Can you work these out from the model? Positions are in its coordinate system, mm. A direction names the side the tool comes from. Coordinates: 2 decimals unless noted, no trailing zeros. Loops run counter-clockwise (first coordinate to the right, second up) from the corner with the lowest first, then second, coordinate; pieces in that order, holes last. Notation, with made-up numbers: (28.25, -37) - (86.25, -37) arc R22 ccw to (86.25, -3) - close; hole circle Ø9 at (-39.5, -12.75). An arc over 180 degrees is marked (long way). Put each result on its own line as item: value. Start each with the question number.
Solid Edge part; units mm, degrees
sketch "Sketch1" plane through (0, 0, 0) normal (0, 0, 1) x (1, 0, 0)
  circle A0 centre (0, 0) radius 10
extrude "Protrusion1" add sketch "Sketch1" along normal mid plane 11
sketch "Sketch2" plane through (0, 0, 5.5) normal (0, 0, 1) x (0, 1, 0)
  circle A0 centre (0, 0) radius 14.5
extrude "ExtrudedProtrusion_2" add sketch "Sketch2" along normal blind 3
mirror "Mirror1" about plane through (0, 0, 0) normal (0, 0, -1) of "ExtrudedProtrusion_2"
sketch "Sketch3" plane through (0, 0, 8.5) normal (0, 0, 1) x (0, -1, 0)
  line L0 (3.9285, -6.3953) -> (7.5028, 0.2046)
  line L1 (7.5028, 0.2046) -> (3.5742, 6.5999)
  line L2 (3.5742, 6.5999) -> (-3.9285, 6.3953)
  line L3 (-3.9285, 6.3953) -> (-7.5028, -0.2046)
  line L4 (-7.5028, -0.2046) -> (-3.5742, -6.5999)
  line L5 (-3.5742, -6.5999) -> (3.9285, -6.3953)
extrude "ExtrudedCutout_1" cut sketch "Sketch3" against normal blind 37.5006
properties part number "BumbleB0195"
Q1. On a 3-axis mill with a long thin cutter (end or side, diameter ignored), from which of +Z, -Z, +X, -X, +Y, -Y can I reach the whole of each face in a straight line? I mean faces 5 (the flat face through (-3, 10, -5.5)), 6 (the flat face through (-3.14, -5.69, 0.12)), 7 (the flat face through (7, 0, -8.5)). Say none if no direction works.
Q2. I want a section at B-B on z = 4.75. List the corners of the cut face in (x, y) for me.
Q3. Will these pins go through, and if not, where does the flat tip stop? pin 1 (1 mm diameter, centred on x = 3.5, z = -3.5, fed in from +Y); pin 2 (1.5 mm diameter, centred on x = 9.5, z = 1, fed in from +Y); pin 3 (10 mm diameter, centred on x = 6, z = 5.5, fed in from -Y); pin 4 (8.5 mm diameter, centred on x = -1, y = -3, fed in from +Z).
Q4. We'd pull the mould along Z, two halves only. Please class faces 1 (the flat face through (3, 10, 5.5)), 2 (the flat face through (3.14, 5.69, 0.12)), 3 (the cylindrical face through (-2.17, -9.76, 0.08)), 4 (the flat face through (-7, 0, 8.5)): released by +Z, released by -Z, zero draft, split by the parting line, or undercut.
Q5. Please list where these lines run through material, in increasing order: line 1 along Z through (x, y) = (-10.75, 6); line 2 along X through (y, z) = (7.25, -0.5); line 3 along Y through (x, z) = (4.5, -4). Write a range as [from, to].
Q6. I want a section at D-D on x = -8.25. List the corners of the cut face in (y, z) for me.
Q7. I want a section at C-C on y = 1.5. List the corners of the cut face in (x, z) for me, and give its area (3 significant figures).
Q8. I want a section at A-A on x = 10.5. List the corners of the cut face in (y, z) for me.
Calculated:
1. face 5: none
1. face 6: +Z, -Z
1. face 7: -Z, +X, -X, +Y, -Y
2. outline: circle Ø20 at (0, 0); hole (-6.6, 3.57) - (-6.4, -3.93) - (0.2, -7.5) - (6.6, -3.57) - (6.4, 3.93) - (-0.2, 7.5) - close
3. pin 1: y = 9.54
3. pin 2: y = 4.84
3. pin 3: y = -14.47
3. pin 4: z = 8.5
4. face 1: undercut
4. face 2: zero draft
4. face 3: undercut
4. face 4: released by +Z
5. line 1: [-8.5, -5.5], [5.5, 8.5]
5. line 2: [-6.89, -0.62], [0.26, 6.89]
5. line 3: [-8.93, -4.86], [4.95, 8.93]
6. outline: (-11.92, -8.5) - (11.92, -8.5) - (11.92, -5.5) - (5.65, -5.5) - (5.65, 5.5) - (11.92, 5.5) - (11.92, 8.5) - (-11.92, 8.5) - (-11.92, 5.5) - (-5.65, 5.5) - (-5.65, -5.5) - (-11.92, -5.5) - close
7. outline: (-14.42, -8.5) - (-6.54, -8.5) - (-6.54, 8.5) - (-14.42, 8.5) - (-14.42, 5.5) - (-9.89, 5.5) - (-9.89, -5.5) - (-14.42, -5.5) - close; (6.46, -8.5) - (14.42, -8.5) - (14.42, -5.5) - (9.89, -5.5) - (9.89, 5.5) - (14.42, 5.5) - (14.42, 8.5) - (6.46, 8.5) - close
7. area: 169 mm2
8. outline: (-10, -8.5) - (10, -8.5) - (10, -5.5) - (-10, -5.5) - close; (-10, 5.5) - (10, 5.5) - (10, 8.5) - (-10, 8.5) - close
